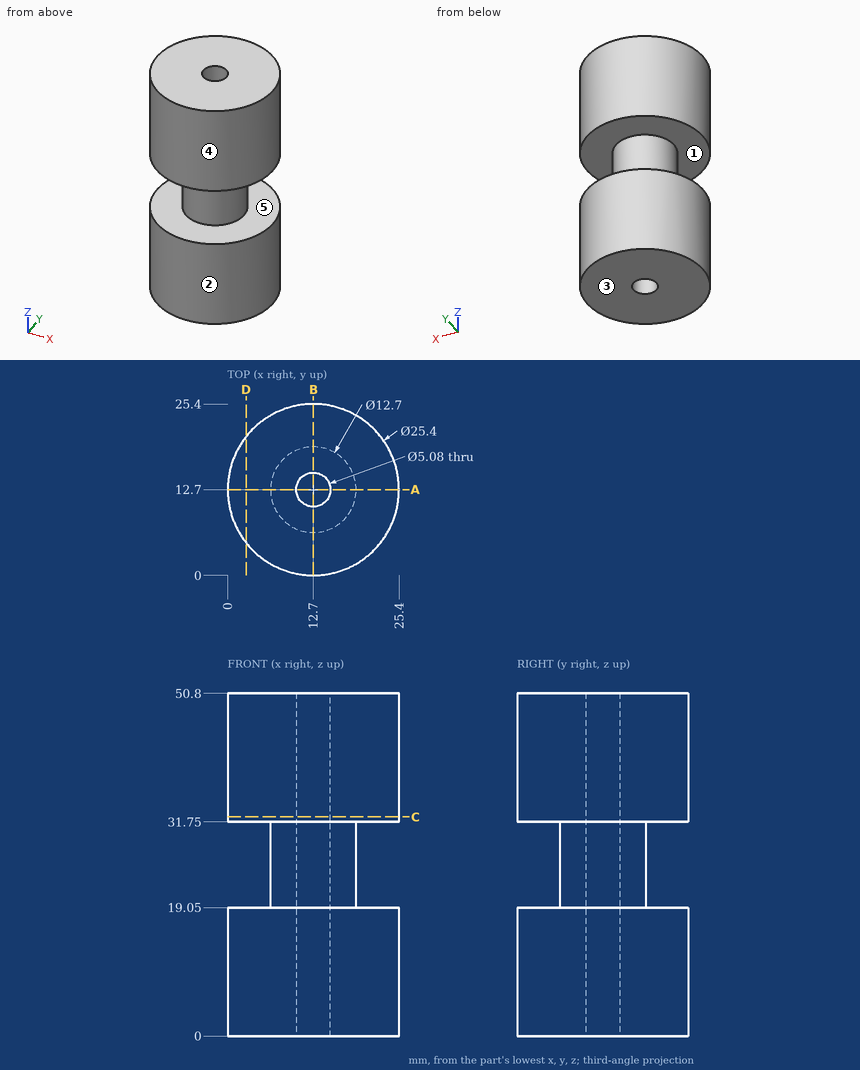
Source: three-view drawing plus pictorial views. Frame: mm from the lowest corner of the part. A direction names the side the tool comes from. Coordinates: 2 decimals unless noted, no trailing zeros. Order: outer loops, then holes, each group sorted by start corner. A loop starts at its lowest first (then second) coordinate and runs counter-clockwise, first axis right, second up. Notation, with made-up numbers: M 86,-15.5 L 110,-15.5 A13 ccw 110,2.5 Z; hole C -1.5,24 d3. An arc over 180 degrees is marked long. One line per question, with ' | ' between items. Start each with the question number.
Item 1: Pin query (flat end, axial travel): pin 1 Ø1 at (x, z) = (13.5, 24.5) entering from +Y; pin 2 Ø2 at (x, z) = (3, 42.5) entering from -Y; pin 3 Ø1.5 at (x, z) = (18.5, 17.5) entering from +Y. Return the tip coordinate at first contact, or that it passes through.
Item 2: Draft query along Z for the marked faces 3, 4 and 5. Return one class per face: released by +Z, released by -Z, zero draft, split by the parting line, or undercut.
Item 3: Cut plane A-A, the plane y = 12.7. Return the cut outline in (x, z), then the cut area to 3 significant figures.
Item 4: Set-up query: the marked faces 1 and 2. Return all of +Z, -Z, +X, -X, +Y, -Y with unobstructed straight access to the full face (end or side cutting, diameter ignored); none if empty.
Item 5: Cut plane D-D, the plane x = 2.75. Return the cut outline in (y, z).
Item 6: Cut plane C-C, the plane z = 32.5. Return the cut outline in (x, y), then the cut area to 3 significant figures.
Item 7: Ray query, probe 1 along Z at (x, y) = (20, 10.75); probe 2 along Y at (x, z) = (12.7, 28.5); probe 3 along Y at (x, z) = (12.7, 39). Return the intervals inside material, ascending. Write a range as [from, to].
A:
1) pin 1: stops at y = 19.04 | pin 2: stops at y = 3.45 | pin 3: stops at y = 24.35
2) face 3: released by -Z | face 4: zero draft | face 5: undercut
3) outline: M 0,0 L 10.16,0 L 10.16,50.8 L 0,50.8 L 0,31.75 L 6.35,31.75 L 6.35,19.05 L 0,19.05 Z; M 15.24,0 L 25.4,0 L 25.4,19.05 L 19.05,19.05 L 19.05,31.75 L 25.4,31.75 L 25.4,50.8 L 15.24,50.8 Z | area: 871 mm2
4) face 1: none | face 2: +Z, -Z
5) outline: M 4.81,0 L 20.59,0 L 20.59,19.05 L 4.81,19.05 Z; M 4.81,31.75 L 20.59,31.75 L 20.59,50.8 L 4.81,50.8 Z
6) outline: C 12.7,12.7 d25.4; hole C 12.7,12.7 d5.08 | area: 486 mm2
7) probe 1: z = [0, 19.05], [31.75, 50.8] | probe 2: y = [6.35, 10.16], [15.24, 19.05] | probe 3: y = [0, 10.16], [15.24, 25.4]
